Here's the drawing with two shaded views (mm, measured from the low corner). I have some questions. Give positions to 0.01 mm unless a question says otherwise; leave off trailing zeros. Write each loop counter-clockwise with the first axis right and the second up, starting at its lowest first coordinate (ties: lowest second). Pieces come first, ordered by that corner, then holes. Notation, with made-up numbers: (43.5, -39) - (86.5, -39) arc R20 ccw to (86.5, -21) - close; hole circle Ø2 at (42.25, 77). An arc over 180 degrees is marked (long way). Answer as CSV lines item,"result". Start each with the question number.
Q1. Will these pins go through, and if not, where does the flat tip stop? pin 1 Ø6 at (y, z) = (22.5, 10) entering from -X; pin 2 Ø1.5 at (x, y) = (8, 69) entering from -Z; pin 3 Ø5 at (y, z) = (44.5, 4) entering from +X.
Q2. If I drill on line 1 along Y through (x, z) = (3.5, 11.5) (3 decimals); line 2 along Z through (x, y) = (6.25, 15), over which ranges is the centre line in solid material (lowest first)?
Q3. We'd pull the mould along Y, two halves only. Please class the marked faces 1, 2 and 3: pulls with the +Y half, pulls with the -Y half, needs draft (parallel to the pull), parting line crosses it, or undercut.
Q4. Imagine slicing it at C-C on y = 38. List the corners of the cut face in (x, z) for me.
Q5. Imagine slicing it at B-B on z = 6.35. List the corners of the cut face in (x, y) for me (3 decimals).
Q6. Imagine slicing it at A-A on x = 6.35. List the corners of the cut face in (y, z) for me (3 decimals), and give its area (3 significant figures).
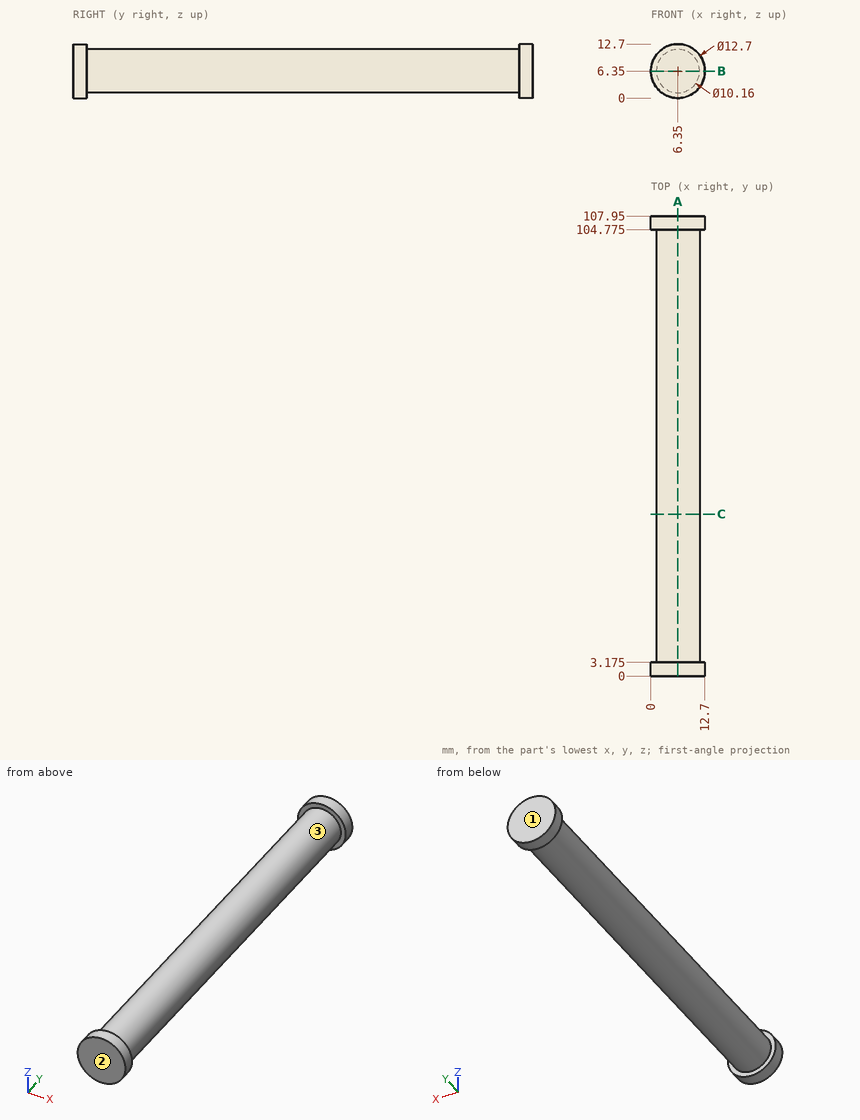
Conclusion:
1,pin 1,"x = 1.31"
1,pin 2,"z = 1.35"
1,pin 3,"x = 11.43"
2,line 1,"0 to 3.175, 104.775 to 107.95"
2,line 2,"1.27 to 11.43"
3,face 1,"pulls with the +Y half"
3,face 2,"pulls with the -Y half"
3,face 3,"undercut"
4,outline,"circle Ø10.16 at (6.35, 6.35)"
5,outline,"(0, 0) - (12.7, 0) - (12.7, 3.175) - (11.43, 3.175) - (11.43, 104.775) - (12.7, 104.775) - (12.7, 107.95) - (0, 107.95) - (0, 104.775) - (1.27, 104.775) - (1.27, 3.175) - (0, 3.175) - close"
6,outline,"(0, 0) - (3.175, 0) - (3.175, 1.27) - (104.775, 1.27) - (104.775, 0) - (107.95, 0) - (107.95, 12.7) - (104.775, 12.7) - (104.775, 11.43) - (3.175, 11.43) - (3.175, 12.7) - (0, 12.7) - close"
6,area,"1,110 mm^2"
